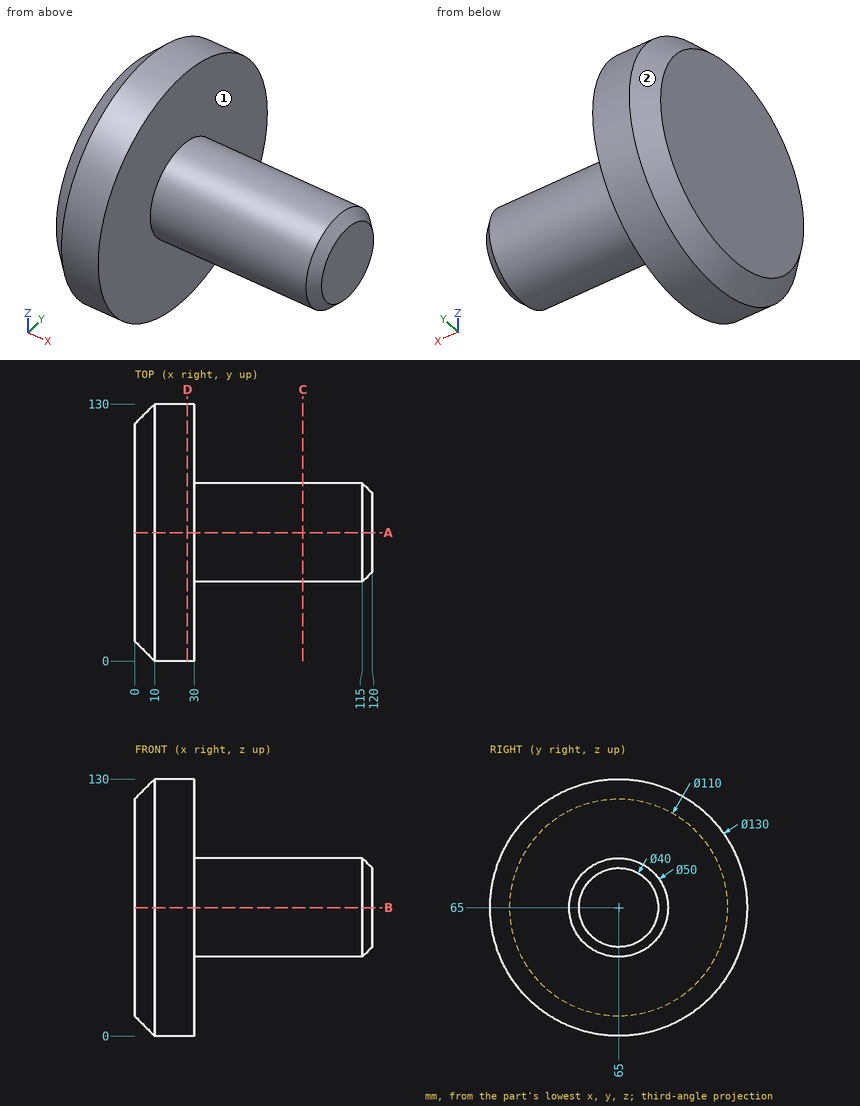
Could you check a few things on this drawing? It's one solid part, dimensions in mm from its lowest x, y, z. A direction names the side the tool comes from. Round coordinates to 2 decimals unless told otherwise and drop trailing zeros. Loops run counter-clockwise (first coordinate to the right, second up) from the corner with the lowest first, then second, coordinate; pieces in that order, holes last. Notation, with made-up numbers: M -25,83.5 L 4,83.5 A25 ccw 4,119.5 Z; hole C -9.5,-23.5 d8. An arc over 180 degrees is marked long. Write item = value, one per line. Start each with the question number.
(1) Suppose I cut it at A-A on y = 65. Write out the boundary of the cut face in (x, z).
(2) Suppose I cut it at D-D on x = 26.5. Write out the boundary of the cut face in (y, z).
(3) I need wall thicknesses on line 1 along X through (y, z) = (85.5, 87); line 2 along Z through (x, y) = (28, 76.5); line 3 along X through (y, z) = (22.5, 19). Which ranges of each line are inside material? Lowest first, please.
(4) Which directions (+Z, -Z, +X, -X, +Y, -Y) give clear straight access to the entire face, cutting with the end or side of a thin tool? Please do the marked faces 1 and 2.
(5) I'm going to push flat-ended pins straight in: P1, Ø10, axis at y = 53, z = 107, coming from the +X side; P2, Ø1.5, axis at x = 98, z = 80.5, coming from the -Y side; P3, Ø12, axis at x = 78, y = 67, coming from the -Z side. Where does each tip first touch, or does it pass through?
(6) Suppose I cut it at C-C on x = 85. Write out the boundary of the cut face in (y, z).
Answer block:
q1.outline = M 0,10 L 10,0 L 30,0 L 30,40 L 115,40 L 120,45 L 120,85 L 115,90 L 30,90 L 30,130 L 10,130 L 0,120 Z
q2.outline = C 65,65 d130
q3.line_1 = 0 to 30
q3.line_2 = 1.03 to 128.97
q3.line_3 = 7.63 to 30
q4.face_1 = +X
q4.face_2 = -X
q5.P1 = 30
q5.P2 = 44.81
q5.P3 = 40
q6.outline = C 65,65 d50
